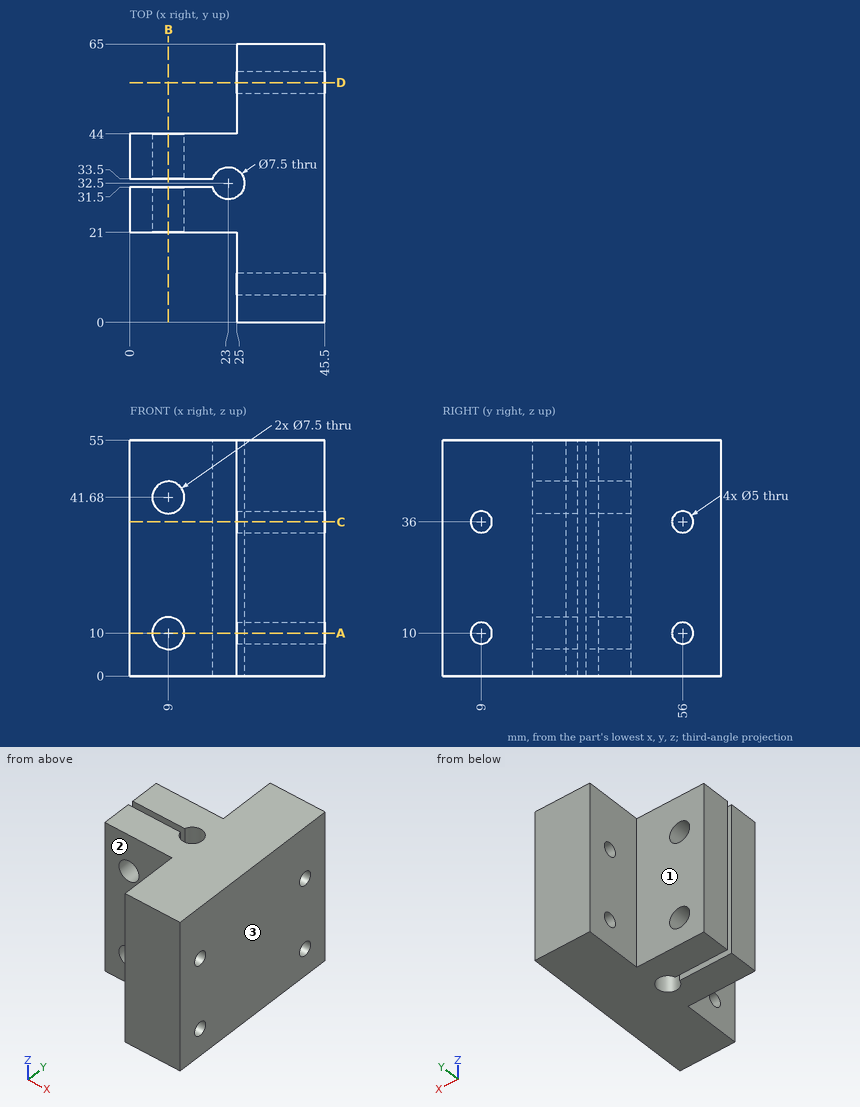
Design review of the part shown in the three views and the two pictorial views. Dimensions are in mm from the part's minimum x, y and z. A direction names the side the tool comes from. Coordinates: 2 decimals unless noted, no trailing zeros. Loops run counter-clockwise (first coordinate to the right, second up) from the corner with the lowest first, then second, coordinate; pieces in that order, holes last. Notation, with made-up numbers: (14, -31.5) - (53, -31.5) arc R17 cw to (53, -24.5) - close; hole circle Ø7 at (25, 20.5). An arc over 180 degrees is marked (long way). Use a Markdown table: item, result. Add a question column.
Item 1: We need section B-B (x = 9). Give the boundary of the cut face in (y, z), and give its area (3 significant figures).
Item 2: We need section D-D (y = 56). Give the boundary of the cut face in (x, z), and give its area (4 significant figures).
Item 3: We need section C-C (z = 36). Give the boundary of the cut face in (x, y).
Item 4: Tool access review of the marked faces 1, 2 and 3: name each direction out of +Z, -Z, +X, -X, +Y, -Y from which nothing blocks a thin tool from reaching the whole face with its end or side.
Item 5: Insertion check: pin 1 Ø1 at (y, z) = (19, 38.5) entering from -X; pin 2 Ø8.5 at (x, z) = (9, 10) entering from -Y; pin 3 Ø6 at (x, z) = (10, 27.5) entering from +Y; pin 4 Ø8 at (x, z) = (35.5, 36) entering from -Y. Each pin has a flat end and moves straight along its axis. Give the tip position at first contact, or say it passes through.
Item 6: For line 1 (Y direction, x = 13.5, z = 20.5); line 2 (Z direction, x = 28, y = 9); line 3 (Z direction, x = 9, y = 27), list the stretches that pass through material, from the lowest coordinate up.
Item 7: We need section A-A (z = 10). Give the boundary of the cut face in (x, y).
Results list:
| question | item | result |
|---|---|---|
| 1 | outline | (21, 0) - (31.5, 0) - (31.5, 6.25) - (21, 6.25) - close; (21, 13.75) - (31.5, 13.75) - (31.5, 37.93) - (21, 37.93) - close; (21, 45.43) - (31.5, 45.43) - (31.5, 55) - (21, 55) - close; (33.5, 0) - (44, 0) - (44, 6.25) - (33.5, 6.25) - close; (33.5, 13.75) - (44, 13.75) - (44, 37.93) - (33.5, 37.93) - close; (33.5, 45.43) - (44, 45.43) - (44, 55) - (33.5, 55) - close |
| 1 | area | 840 mm^2 |
| 2 | outline | (25, 0) - (45.5, 0) - (45.5, 7.5) - (25, 7.5) - close; (25, 12.5) - (45.5, 12.5) - (45.5, 33.5) - (25, 33.5) - close; (25, 38.5) - (45.5, 38.5) - (45.5, 55) - (25, 55) - close |
| 2 | area | 922.5 mm^2 |
| 3 | outline | (0, 21) - (25, 21) - (25, 11.5) - (45.5, 11.5) - (45.5, 53.5) - (25, 53.5) - (25, 44) - (0, 44) - (0, 33.5) - (19.39, 33.5) arc R3.75 cw (long way) to (19.39, 31.5) - (0, 31.5) - close; (25, 0) - (45.5, 0) - (45.5, 6.5) - (25, 6.5) - close; (25, 58.5) - (45.5, 58.5) - (45.5, 65) - (25, 65) - close |
| 4 | face 1 | +Z, -Z, -X, +Y |
| 4 | face 2 | +Z, -Z, -X, -Y |
| 4 | face 3 | +Z, -Z, +X, +Y, -Y |
| 5 | pin 1 | stops at x = 25 |
| 5 | pin 2 | stops at y = 21 |
| 5 | pin 3 | stops at y = 44 |
| 5 | pin 4 | stops at y = 0 |
| 6 | line 1 | y = 21 to 31.5, 33.5 to 44 |
| 6 | line 2 | z = 0 to 7.5, 12.5 to 33.5, 38.5 to 55 |
| 6 | line 3 | z = 0 to 6.25, 13.75 to 37.93, 45.43 to 55 |
| 7 | outline | (0, 21) - (5.25, 21) - (5.25, 31.5) - (0, 31.5) - close; (0, 33.5) - (5.25, 33.5) - (5.25, 44) - (0, 44) - close; (12.75, 21) - (25, 21) - (25, 11.5) - (45.5, 11.5) - (45.5, 53.5) - (25, 53.5) - (25, 44) - (12.75, 44) - (12.75, 33.5) - (19.39, 33.5) arc R3.75 cw (long way) to (19.39, 31.5) - (12.75, 31.5) - close; (25, 0) - (45.5, 0) - (45.5, 6.5) - (25, 6.5) - close; (25, 58.5) - (45.5, 58.5) - (45.5, 65) - (25, 65) - close |
